Check sheet for the drawn part. Datum: minimum x, y, z corner. Units: mm. Round coordinates to 2 decimals unless told otherwise and drop trailing zeros. Write each loop counter-clockwise with the first axis right and the second up, starting at its lowest first coordinate (ties: lowest second). Pieces come first, ordered by that corner, then holes. Notation, with made-up numbers: M 24,59 L 52,59 A22 ccw 52,93 Z; hole C 41,-27 d1. An arc over 180 degrees is marked long. One line per item, written item: value. Start each with the question number.
1. Section check D-D (z = 40). Record the boundary of the cut face in (x, y).
2. Scan lines: probe 1 along Z at (x, y) = (134.5, 7.25); probe 2 along Y at (x, z) = (41, 161.5). Record each from-to range of solid material in increasing order. Write a range as [from, to].
3. Section check B-B (y = 8). Record the boundary of the cut face in (x, z).
4. Section check C-C (x = 48). Record the boundary of the cut face in (y, z) (1 decimal), and give its area (3 significant figures).
5. Depth check by flat-ended pin: P1, Ø5, axis at x = 90.5, y = 7.5, coming from the +Z side; P2, Ø3, axis at x = 75, y = 5.5, coming from the +Z side; P3, Ø2.5, axis at y = 8, z = 341.5, coming from the -X side. Enter the tip coordinate at first touch or a pass-through.
6. Section check A-A (z = 542.5). Record the boundary of the cut face in (x, y), and give its area (3 significant figures).
7. Release check for a two-part mould opening along Z. For the marked faces 1 and 2 record: pulls with the +Z half, pulls with the -Z half, needs draft (parallel to the pull), parting line crosses it, or undercut.
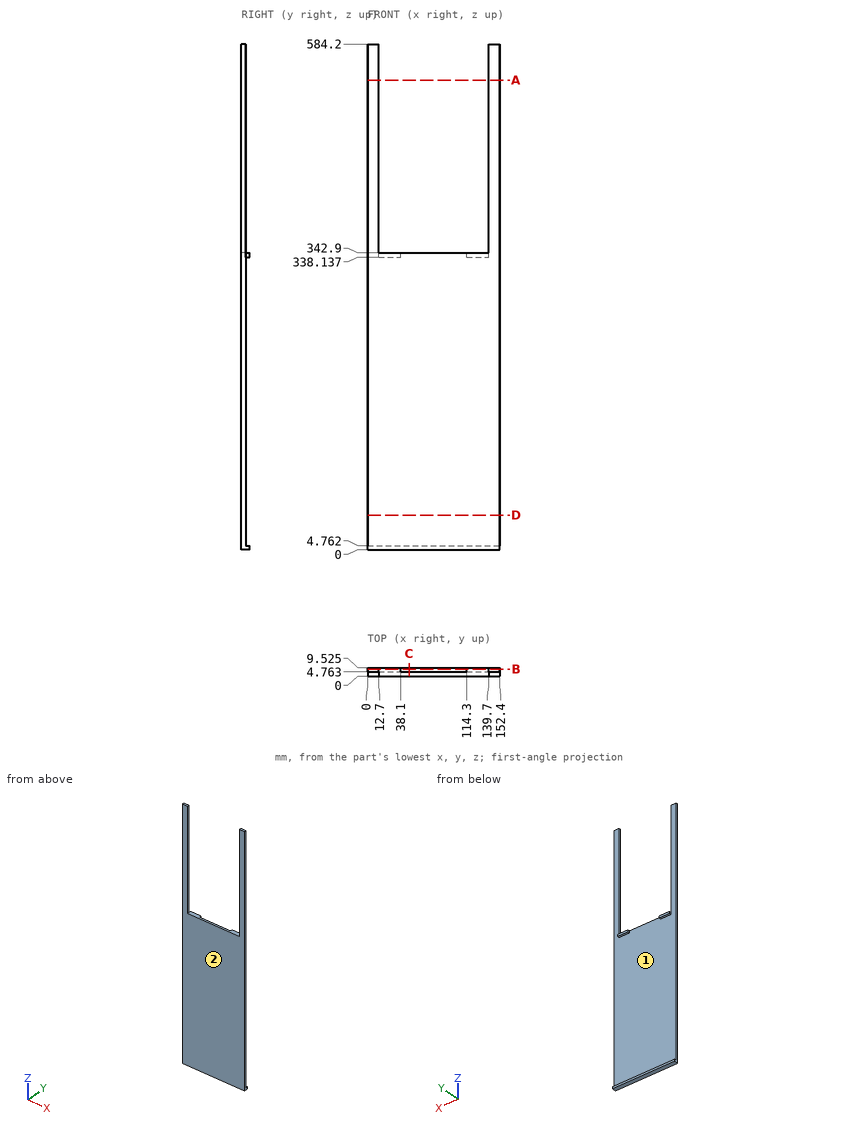
Result sheet:
1. outline: M 0,0 L 152.4,0 L 152.4,4.76 L 0,4.76 Z
2. probe 1: z = [0, 4.76], [338.14, 342.9]
2. probe 2: y = [0, 4.76]
3. outline: M 0,0 L 152.4,0 L 152.4,4.76 L 0,4.76 Z; M 12.7,338.14 L 38.1,338.14 L 38.1,342.9 L 12.7,342.9 Z; M 114.3,338.14 L 139.7,338.14 L 139.7,342.9 L 114.3,342.9 Z
4. outline: M 0,0 L 9.5,0 L 9.5,4.8 L 4.8,4.8 L 4.8,342.9 L 0,342.9 Z
4. area: 1,660 mm2
5. P1: stops at z = 4.76
5. P2: stops at z = 342.9
5. P3: stops at x = 12.7
6. outline: M 0,0 L 12.7,0 L 12.7,4.76 L 0,4.76 Z; M 139.7,0 L 152.4,0 L 152.4,4.76 L 139.7,4.76 Z
6. area: 121 mm2
7. face 1: undercut
7. face 2: needs draft
